Read the model definition and answer for the solid it produces. Units are mm, in the model's axes. Face numbers are marked on the shaded views. A direction names the side the tool comes from. Coordinates: 2 decimals unless noted, no trailing zeros. Write each loop counter-clockwise with the first axis right and the second up, starting at its lowest first coordinate (ties: lowest second). Pieces come first, ordered by that corner, then holes. Notation, with made-up numbers: (-9, -10) -> (48, -10) arc R34 ccw to (48, 20) -> close; hole circle Ø9 at (-29.75, -11). An arc over 180 degrees is marked (long way). One line per item, written item: value. Start each with the question number.
1. For the marked faces 4, 5, 6 and 7, determine the directions among +Z, -Z, +X, -X, +Y, -Y from which every point of the face is accessible in a straight line to the end or side of a thin tool.
2. Given P1, Ø3.5, axis at y = 0.5, z = 3.5, coming from the -X side, flat-ended and moving along its own axis, determine where the tip first touches the part or whether it passes through.
3. Find section A-A, the plane x = -3.61. Write down the section's boundary in (y, z).
4. Consider line 1 along Y through (x, z) = (-3.5, 4); line 2 along Y through (x, z) = (24.39, 4); line 3 along Y through (x, z) = (10.39, 4). Determine where each line is inside the solid, lowest interval first.
5. Find section B-B, the plane y = 14. Write down the section's boundary in (x, z), and give its area (3 significant figures).
6. Find section D-D, the plane y = -14. Write down the section's boundary in (x, z), and give its area (3 significant figures).
7. Find section C-C, the plane x = 24.39. Write down the section's boundary in (y, z).
8. For a pull along Y with two mould halves and no side action, classify the marked faces 1, 2 and 3 as pulls with the +Y half, pulls with the -Y half, needs draft (parallel to the pull), parting line crosses it, or undercut.
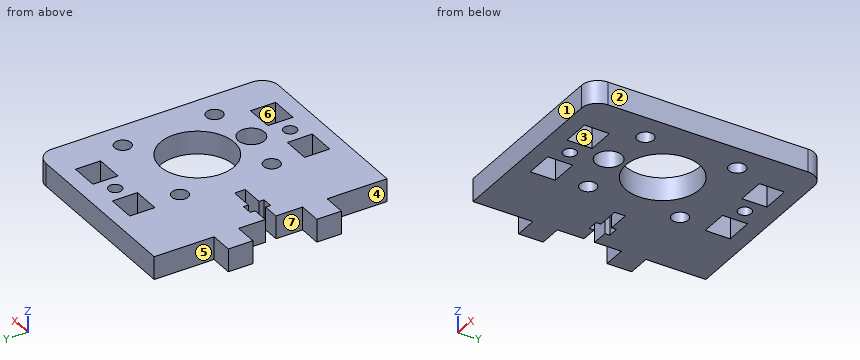
```python
from build123d import *

# Parameters (mm, degrees)
F0_W      = 65
F0_H      = 71
F0_W_2    = 8.5
F0_H_2    = 7.65
F2_DEPTH  = 7
F1_R      = 4
F1_R_2    = 11.25
F1_R_3    = 2.5
F3_DEPTH  = 25
F4_R      = 2
F5_DEPTH  = 7.001
F6_W      = 7
F6_H      = 18.25
F6_H_2    = 19.5
F7_DEPTH  = 7.001
F8_W      = 30
F8_H      = 3.25
F9_W      = 3.25
F9_H      = 6.25
F10_DEPTH = 7.001
F11_R     = 5


with BuildPart() as f2:
    # F0 (on Top) → F2 (new body)
    with BuildSketch(Plane.XY):
        Rectangle(F0_W, F0_H)
        with Locations((-1.25, -26.675)):
            Rectangle(F0_W_2, F0_H_2, mode=Mode.SUBTRACT)
        with Locations((16.75, -26.675)):
            Rectangle(F0_W_2, F0_H_2, mode=Mode.SUBTRACT)
        with Locations((-1.25, 26.675)):
            Rectangle(F0_W_2, F0_H_2, mode=Mode.SUBTRACT)
        with Locations((16.75, 26.675)):
            Rectangle(F0_W_2, F0_H_2, mode=Mode.SUBTRACT)
    extrude(amount=F2_DEPTH)

    # F1 (on face) → F3 (cut)
    with BuildSketch(Plane.XY):
        with Locations((10.39, -16.5)):
            Circle(F1_R)
        with Locations((10.39, 0)):
            Circle(F1_R_2)
        with Locations((-3.61, 14)):
            Circle(F1_R_3)
        with Locations((24.39, 14)):
            Circle(F1_R_3)
        with Locations((24.39, -14)):
            Circle(F1_R_3)
        with Locations((-3.61, -14)):
            Circle(F1_R_3)
    extrude(amount=F3_DEPTH, mode=Mode.SUBTRACT)

    # F4 (on face) → F5 (cut, through all)
    with BuildSketch(Plane.XY.offset(7)):
        with Locations((7.75, 26.675)):
            Circle(F4_R)
        with Locations((7.75, -26.675)):
            Circle(F4_R)
    extrude(amount=-F5_DEPTH, mode=Mode.SUBTRACT)

    # F6 (on face) → F7 (cut, through all)
    with BuildSketch(Plane.XY.offset(7)):
        with Locations((-29, 26.375)):
            Rectangle(F6_W, F6_H)
        with Locations((-29, -26.375)):
            Rectangle(F6_W, F6_H)
        with Locations((-29, 0)):
            Rectangle(F6_W, F6_H_2)
    extrude(amount=-F7_DEPTH, mode=Mode.SUBTRACT)

    # F8 (on face) + F9 (on face) → F10 (cut, through all)
    with BuildSketch(Plane.XY.offset(7)):
        with Locations((-25.5, 0)):
            Rectangle(F8_W, F8_H)
    with BuildSketch(Plane.XY.offset(7)):
        with Locations((-18.875, 0)):
            Rectangle(F9_W, F9_H)
    extrude(amount=-F10_DEPTH, mode=Mode.SUBTRACT)

    # F11
    f11_edges = [f2.edges().sort_by_distance(p)[0] for p in [
        (32.5, -35.5, 3.5),
        (32.5, 35.5, 3.5),
    ]]
    fillet(f11_edges, radius=F11_R)


solid = f2.part
```
Answer block:
1. face 4: +Z, -Z, -X, -Y
1. face 5: +Z, -Z, -X, +Y
1. face 6: +Z, -Z
1. face 7: +Z, -Z, -X
2. P1: stops at x = -25.5
3. outline: (-35.5, 0) -> (-30.5, 0) -> (-30.5, 7) -> (-35.5, 7) -> close; (-22.85, 0) -> (-16.5, 0) -> (-16.5, 7) -> (-22.85, 7) -> close; (-11.5, 0) -> (11.5, 0) -> (11.5, 7) -> (-11.5, 7) -> close; (16.5, 0) -> (22.85, 0) -> (22.85, 7) -> (16.5, 7) -> close; (30.5, 0) -> (35.5, 0) -> (35.5, 7) -> (30.5, 7) -> close
4. line 1: y = -35.5 to -30.5, -22.85 to -16.5, -11.5 to 11.5, 16.5 to 22.85, 30.5 to 35.5
4. line 2: y = -35.5 to -16.5, -11.5 to 11.5, 16.5 to 35.5
4. line 3: y = -35.5 to -20.5, -12.5 to -11.25, 11.25 to 35.5
5. outline: (-32.5, 0) -> (-6.11, 0) -> (-6.11, 7) -> (-32.5, 7) -> close; (-1.11, 0) -> (21.89, 0) -> (21.89, 7) -> (-1.11, 7) -> close; (26.89, 0) -> (32.5, 0) -> (32.5, 7) -> (26.89, 7) -> close
5. area: 385 mm2
6. outline: (-32.5, 0) -> (-6.11, 0) -> (-6.11, 7) -> (-32.5, 7) -> close; (-1.11, 0) -> (7.27, 0) -> (7.27, 7) -> (-1.11, 7) -> close; (13.51, 0) -> (21.89, 0) -> (21.89, 7) -> (13.51, 7) -> close; (26.89, 0) -> (32.5, 0) -> (32.5, 7) -> (26.89, 7) -> close
6. area: 341 mm2
7. outline: (-35.5, 0) -> (-16.5, 0) -> (-16.5, 7) -> (-35.5, 7) -> close; (-11.5, 0) -> (11.5, 0) -> (11.5, 7) -> (-11.5, 7) -> close; (16.5, 0) -> (35.5, 0) -> (35.5, 7) -> (16.5, 7) -> close
8. face 1: pulls with the -Y half
8. face 2: needs draft
8. face 3: undercut
